Check sheet for the modelled part. Datum: model origin and axes. Units: mm. A direction names the side the tool comes from. Give positions to 0.01 mm unless a question says otherwise; leave off trailing zeros. Write each loop counter-clockwise with the first axis right and the second up, starting at its lowest first coordinate (ties: lowest second). Pieces come first, ordered by that corner, then holes. Notation, with made-up numbers: M 47.25,73.25 L 61.25,73.25 A15 ccw 61.25,96.25 Z; hole C 47.5,-15 d5. An arc over 180 degrees is marked long. Write item = value, one per line. Start each with the question number.
1) Cross-section at A-A, the plane y = -9. Record the cut outline in (x, z) (3 decimals).
2) Scan lines: line 1 along Z through (x, y) = (0, -9.25) (3 decimals); line 2 along X through (y, z) = (-3.5, -12); line 3 along Z through (x, y) = (-5.5, -7.75). Record each from-to range of solid material in increasing order. Write a range as [from, to].
3) Access from +Z, -Z, +X, -X, +Y, -Y to the whole of each face (thin tool, end or side, straight path). Record for faces 1 (the cylindrical face through (-8.948, -9.569, 40.293)), 2 (the flat face through (-10, 6.35, 9)), 3 (the cylindrical face through (-7.559, -0.178, 5.796)).
4) Go/stop test with flat-tipped pins: pin 1 (2 mm diameter, centred on x = -5, y = 0.5, fed in from +Z); pin 2 (15 mm diameter, centred on x = -24.75, z = 14.29, fed in from +Y); pin 3 (11 mm diameter, centred on x = 0, z = -28.575, fed in from -Y). Record where each tip stops, or that it passes through.
5) Cross-section at C-C, the plane y = 2.5. Give the number of separate pieces and of enclosed holes in the cut face, plus the area to 3 significant figures.
6) Mould release check, pull along Y, two halves, no side actions. Record for faces 4 (the conical face through (-30.724, 0.255, -23.558)), 5 (the flat face through (0, 12.7, 42)), 6 (the flat face through (-10, -6.35, 9)): released by +Y, released by -Y, zero draft, split by the parting line, or undercut.
```python
from build123d import *

# Parameters (mm, degrees)
SKETCH2_R          = 41.275
SKETCH2_R_2        = 12.7
CUT_EXTRUDE1_DEPTH = 6.35
SKETCH3_R          = 9.525
CUT_EXTRUDE2_DEPTH = 13.7
SKETCH5_R          = 4.7625
CUT_EXTRUDE3_DEPTH = 7.35
CIRPATTERN1_COUNT  = 6


with BuildPart() as part:
    # Sketch1 → Revolve1 (revolve)
    with BuildSketch(Plane.XY):
        Polygon((0, 0), (0, 12.7), (50.8, 12.7), (50.8, 5.260512242), (38.1, 0), align=None)
    revolve(axis=Axis((0, 218.832128387, 0), (0, -1, 0)))

    # Sketch2 → Cut-Extrude1 (cut)
    with BuildSketch(Plane(origin=(0, 12.7, 0), x_dir=(1, 0, 0), z_dir=(0, 1, 0))):
        Circle(SKETCH2_R)
        Circle(SKETCH2_R_2, mode=Mode.SUBTRACT)
    extrude(amount=-CUT_EXTRUDE1_DEPTH, mode=Mode.SUBTRACT)

    # Sketch3 → Cut-Extrude2 (cut, through all)
    with BuildSketch(Plane(origin=(0, 12.7, 0), x_dir=(1, 0, 0), z_dir=(0, 1, 0))):
        Circle(SKETCH3_R)
    extrude(amount=-CUT_EXTRUDE2_DEPTH, mode=Mode.SUBTRACT)

    # Sketch5 → Cut-Extrude3 (cut, through all)
    with BuildSketch(Plane(origin=(0, 6.35, 0), x_dir=(1, 0, 0), z_dir=(0, 1, 0))):
        with Locations((0, 28.575)):
            Circle(SKETCH5_R)
    cut_extrude3 = extrude(amount=-CUT_EXTRUDE3_DEPTH, mode=Mode.SUBTRACT)

    # CirPattern1: Cut-Extrude3 ×6 about axis
    cirpattern1_axis = Axis((0, 0, 0), (0, 1, 0))
    for i in range(1, CIRPATTERN1_COUNT):
        add(cut_extrude3.rotate(cirpattern1_axis, i * 360 / CIRPATTERN1_COUNT), mode=Mode.SUBTRACT)

    # Mirror1: part across plane


with BuildPart() as part_1:
    add(part.part)
    add(part.part.mirror(Plane.ZX))


solid = part_1.part
```
Reply:
q1.outline = C 0,0 d101.6; C 0,0 d25.4; hole C 0,0 d82.55; hole C 0,0 d19.05
q2.line_1 = [-50.8, -41.275], [-12.7, -9.525], [9.525, 12.7], [41.275, 50.8]
q2.line_2 = [-44.98, -28.92], [-20.57, 20.57], [28.92, 44.98]
q2.line_3 = [-50.5, -40.91], [-11.45, -7.78], [7.78, 11.45], [40.91, 50.5]
q3.face_1 = -Y
q3.face_2 = +Y
q3.face_3 = +Y, -Y
q4.pin_1 = 41.42
q4.pin_2 = 6.35
q4.pin_3 = -6.35
q5.separate_pieces = 1
q5.enclosed_holes = 7
q5.area = 5,410 mm2
q6.face_4 = undercut
q6.face_5 = released by +Y
q6.face_6 = released by -Y
